Print and shaded views of the part. All mm, measured from the part's lowest x, y and z. Round coordinates to 2 decimals unless told otherwise and drop trailing zeros. Write each loop counter-clockwise with the first axis right and the second up, starting at its lowest first coordinate (ties: lowest second). Pieces come first, ordered by that corner, then holes. Notation, with made-up numbers: (69.25, 38.5) -> (95.25, 38.5) arc R18 cw to (95.25, 56.5) -> close; hole circle Ø8 at (9, 24.25). An arc over 180 degrees is marked (long way). Return JSON: item names as keys, results as strings. Group by question number.
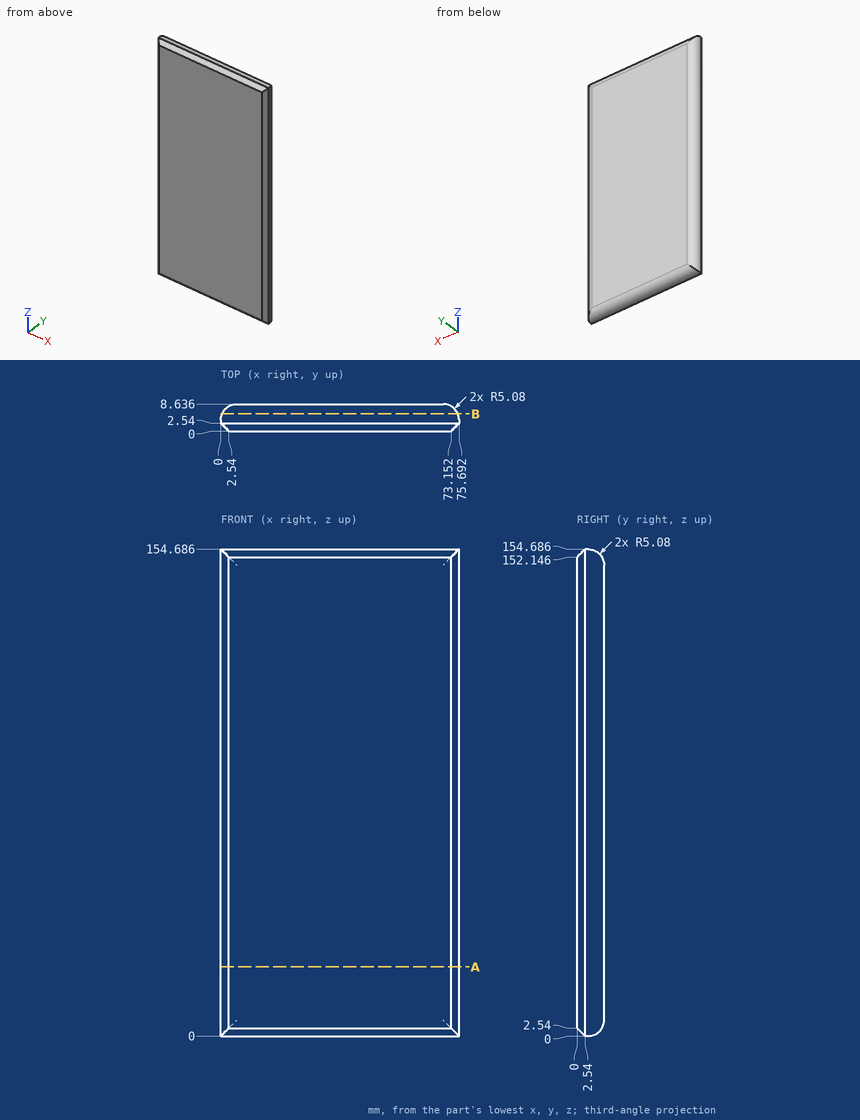
Item 1: Flat gauge pins, fed straight in: P1, Ø4, axis at x = 54, y = 1.5, coming from the +Z side; P2, Ø1.5, axis at x = 46, y = 7.5, coming from the -Z side. Where does each tip first touch, or does it go through?
Item 2: Wall check: L1, parallel to X at y = 4, z = 28.5; L2, parallel to Z at x = 23.5, y = 4; L3, parallel to Z at x = 17, y = 2. Give the ranges that are in metal, low to high.
Item 3: Cut at A-A (z = 22). Write the cut outline in (x, y), then the cut area to 3 significant figures.
Item 4: Cut at B-B (y = 5.5). Write the cut outline in (x, z).
Checks:
{
 "1": {"P1": "stops at z = 154.69", "P2": "stops at z = 1.13"},
 "2": {"L1": "x = 0.02 to 75.67", "L2": "z = 0.02 to 154.67", "L3": "z = 0.54 to 154.15"},
 "3": {"outline": "(0, 2.54) -> (2.54, 0) -> (73.15, 0) -> (75.69, 2.54) -> (75.69, 3.56) arc R5.08 ccw to (70.61, 8.64) -> (5.08, 8.64) arc R5.08 ccw to (0, 3.56) -> close", "area": "636 mm2"},
 "4": {"outline": "(0.39, 0.39) -> (75.31, 0.39) -> (75.31, 154.3) -> (0.39, 154.3) -> close"}
}
